```python
from build123d import *

# Parameters (mm, degrees)
SKETCH1_R           = 55
BOSS_EXTRUDE1_DEPTH = 3
CUT_EXTRUDE1_DEPTH  = 3
SKETCH3_R           = 2.5
CUT_EXTRUDE2_DEPTH  = 2


with BuildPart() as part:
    # Sketch1 → Boss-Extrude1 (new body)
    with BuildSketch(Plane.XY):
        Circle(SKETCH1_R)
    extrude(amount=BOSS_EXTRUDE1_DEPTH)

    # Sketch2 → Cut-Extrude1 (cut)
    with BuildSketch(Plane(origin=(0, 0, 0), x_dir=(-1, 0, 0), z_dir=(0, 0, -1))):
        with BuildLine():
            Line((43.884277794, 18.177463037), (50.813374288, 21.04758878))
            ThreePointArc((50.813374288, 21.04758878), (45.730828677, 30.556362816), (38.890872965, 38.890872965))
            Line((38.890872965, 38.890872965), (43.884277794, 18.177463037))
        make_face()
        with BuildLine():
            Line((33.587572106, 33.587572106), (38.890872965, 38.890872965))
            ThreePointArc((38.890872965, 38.890872965), (30.556362816, 45.730828677), (21.04758878, 50.813374288))
            Line((21.04758878, 50.813374288), (33.587572106, 33.587572106))
        make_face()
        with BuildLine():
            Line((18.177463037, 43.884277794), (21.04758878, 50.813374288))
            ThreePointArc((21.04758878, 50.813374288), (10.729967711, 53.943190422), (0, 55))
            Line((0, 55), (18.177463037, 43.884277794))
        make_face()
        with BuildLine():
            Line((0, 47.5), (0, 55))
            ThreePointArc((0, 55), (-10.729967711, 53.943190422), (-21.04758878, 50.813374288))
            Line((-21.04758878, 50.813374288), (0, 47.5))
        make_face()
        with BuildLine():
            Line((-18.177463037, 43.884277794), (-21.04758878, 50.813374288))
            ThreePointArc((-21.04758878, 50.813374288), (-30.556362816, 45.730828677), (-38.890872965, 38.890872965))
            Line((-38.890872965, 38.890872965), (-18.177463037, 43.884277794))
        make_face()
        with BuildLine():
            Line((-33.587572106, 33.587572106), (-38.890872965, 38.890872965))
            ThreePointArc((-38.890872965, 38.890872965), (-45.730828677, 30.556362816), (-50.813374288, 21.04758878))
            Line((-50.813374288, 21.04758878), (-33.587572106, 33.587572106))
        make_face()
        with BuildLine():
            Line((-43.884277794, 18.177463037), (-50.813374288, 21.04758878))
            ThreePointArc((-50.813374288, 21.04758878), (-53.943190422, 10.729967711), (-55, 0))
            Line((-55, 0), (-43.884277794, 18.177463037))
        make_face()
        with BuildLine():
            ThreePointArc((-55, 0), (-53.943190422, -10.729967711), (-50.813374288, -21.04758878))
            Line((-50.813374288, -21.04758878), (-47.5, 0))
            Line((-47.5, 0), (-55, 0))
        make_face()
        with BuildLine():
            ThreePointArc((-50.813374288, -21.04758878), (-45.730828677, -30.556362816), (-38.890872965, -38.890872965))
            Line((-38.890872965, -38.890872965), (-43.884277794, -18.177463037))
            Line((-43.884277794, -18.177463037), (-50.813374288, -21.04758878))
        make_face()
        with BuildLine():
            ThreePointArc((-38.890872965, -38.890872965), (-30.556362816, -45.730828677), (-21.04758878, -50.813374288))
            Line((-21.04758878, -50.813374288), (-33.587572106, -33.587572106))
            Line((-33.587572106, -33.587572106), (-38.890872965, -38.890872965))
        make_face()
        with BuildLine():
            ThreePointArc((-21.04758878, -50.813374288), (-10.729967711, -53.943190422), (0, -55))
            Line((0, -55), (-18.177463037, -43.884277794))
            Line((-18.177463037, -43.884277794), (-21.04758878, -50.813374288))
        make_face()
        with BuildLine():
            ThreePointArc((0, -55), (10.729967711, -53.943190422), (21.04758878, -50.813374288))
            Line((21.04758878, -50.813374288), (0, -47.5))
            Line((0, -47.5), (0, -55))
        make_face()
        with BuildLine():
            ThreePointArc((21.04758878, -50.813374288), (30.556362816, -45.730828677), (38.890872965, -38.890872965))
            Line((38.890872965, -38.890872965), (18.177463037, -43.884277794))
            Line((18.177463037, -43.884277794), (21.04758878, -50.813374288))
        make_face()
        with BuildLine():
            ThreePointArc((38.890872965, -38.890872965), (45.730828677, -30.556362816), (50.813374288, -21.04758878))
            Line((50.813374288, -21.04758878), (33.587572106, -33.587572106))
            Line((33.587572106, -33.587572106), (38.890872965, -38.890872965))
        make_face()
        with BuildLine():
            ThreePointArc((50.813374288, -21.04758878), (53.943190422, -10.729967711), (55, 0))
            Line((55, 0), (43.884277794, -18.177463037))
            Line((43.884277794, -18.177463037), (50.813374288, -21.04758878))
        make_face()
        with BuildLine():
            Line((50.813374288, 21.04758878), (47.5, 0))
            Line((47.5, 0), (55, 0))
            ThreePointArc((55, 0), (53.943190422, 10.729967711), (50.813374288, 21.04758878))
        make_face()
    extrude(amount=-CUT_EXTRUDE1_DEPTH, mode=Mode.SUBTRACT)

    # Sketch3 → Cut-Extrude2 (cut)
    with BuildSketch(Plane(origin=(0, 0, 0), x_dir=(-1, 0, 0), z_dir=(0, 0, -1))):
        Circle(SKETCH3_R)
    extrude(amount=-CUT_EXTRUDE2_DEPTH, mode=Mode.SUBTRACT)


solid = part.part
```
CAD build for the part. Positions are in the model's coordinates, mm. A direction names the side the tool comes from. Round coordinates to 2 decimals unless told otherwise and drop trailing zeros. Write each loop counter-clockwise with the first axis right and the second up, starting at its lowest first coordinate (ties: lowest second). Pieces come first, ordered by that corner, then holes. Notation, with made-up numbers: (0, -3.5) -> (24, -3.5) arc R6 cw to (24, 2.5) -> close; hole circle Ø3 at (75, -18). An arc over 180 degrees is marked (long way). Answer in a Markdown table with one row per item. Add a question column.
Item 1: Saw through at B-B, the plane x = -35. Write the cut outline in (y, z), then the cut area to 3 significant figures.
Item 2: Which spindle directions (+Z, -Z, +X, -X, +Y, -Y) get a long thin tool onto all of the face, cutting with end or side? Do faces 4 (the face through (-10.67, -49.18, 1.48)), 5 (the face through (0, 51, 1)), 6 (the face through (0.54, -2.44, 0.99)). Say none if no direction does.
Item 3: Drop flat-ended pins along their axis: pin 1 Ø2.5 at (x, y) = (-1, -0.5) entering from -Z; pin 2 Ø1.5 at (x, y) = (-39.5, -32.5) entering from -Z; pin 3 Ø1.5 at (y, z) = (13, 0.5) entering from +X; pin 4 Ø0.9 at (x, z) = (50, 1) entering from -Y. Give the stop position or say it passes through.
Item 4: Saw through at C-C, the plane y = 5. Write the cut outline in (x, z), then the cut area to 3 significant figures.
Item 5: Saw through at D-D, the plane x = 9. Write the cut outline in (y, z), then the cut area to 3 significant figures.
Item 6: Mould opens along Y. For faces 1 (the face through (51, 0, 1)), 2 (the face through (-19.592, 47.3, 1.479)), 3 (the face through (11, 1, 0)) say: pulls with the +Y half, pulls with the -Y half, needs draft (parallel to the pull), parting line crosses it, or undercut.
Item 7: Drill centre lines: line 1 (Y direction, x = 20.5, z = 1.05); line 2 (X direction, y = -13.5, z = 0.6); line 3 (Y direction, x = 5.5, z = 2.35). Where is each one in solid material? Low to high. Write a range as from..to.
Findings below:
| question | item | result |
|---|---|---|
| 1 | outline | (-39.83, 0) -> (-35, 0) -> (-35, 3) -> (-39.83, 3) -> close; (-32.56, 0) -> (35, 0) -> (35, 3) -> (-32.56, 3) -> close |
| 1 | area | 217 mm^2 |
| 2 | face 4 | +Z, -Z, -Y |
| 2 | face 5 | +Z, -Z, +Y |
| 2 | face 6 | -Z |
| 3 | pin 1 | stops at z = 2 |
| 3 | pin 2 | passes through |
| 3 | pin 3 | stops at x = 47.51 |
| 3 | pin 4 | stops at y = -20.9 |
| 4 | outline | (-48.29, 0) -> (51.94, 0) -> (51.94, 3) -> (-48.29, 3) -> close |
| 4 | area | 301 mm^2 |
| 5 | outline | (-49.5, 0) -> (48.92, 0) -> (48.92, 3) -> (-49.5, 3) -> close |
| 5 | area | 295 mm^2 |
| 6 | face 1 | undercut |
| 6 | face 2 | pulls with the +Y half |
| 6 | face 3 | needs draft |
| 7 | line 1 | y = -49.49..43.32, 49.49..50.73 |
| 7 | line 2 | x = -46.74..49.63 |
| 7 | line 3 | y = -51.64..48.37 |
